from build123d import *

# Parameters (mm, degrees)
CUT_EXTRUDE1_DEPTH = 1.5


with BuildPart() as part:
    # Sketch1 → Revolve1 (revolve)
    with BuildSketch(Plane.XY):
        with BuildLine():
            Line((42.2, 0), (42.2, 1.61))
            Line((42.2, 1.61), (41.81, 2))
            Line((41.81, 2), (2.2, 2))
            Line((2.2, 2), (2.2, 3.8))
            Line((2.2, 3.8), (1.82, 3.8))
            ThreePointArc((1.82, 3.8), (0.762013659, 2.991755338), (0, 1.9))
            Line((0, 1.9), (0, 0))
            Line((0, 0), (42.2, 0))
        make_face()
    revolve(axis=Axis((42.2, 0, 0), (-1, 0, 0)))

    # Sketch2 → Cut-Extrude1 (cut)
    with BuildSketch(Plane.ZY):
        Polygon((-1.25, 0.721687836), (-1.25, -0.721687836), (0, -1.443375673), (1.25, -0.721687836), (1.25, 0.721687836), (0, 1.443375673), align=None)
    extrude(amount=-CUT_EXTRUDE1_DEPTH, mode=Mode.SUBTRACT)


solid = part.part
Model file for the job. Use its own axes, mm. A direction names the side the tool comes from. Give positions to 0.01 mm unless a question says otherwise; leave off trailing zeros. Order: outer loops, then holes, each group sorted by start corner. A loop starts at its lowest first (then second) coordinate and runs counter-clockwise, first axis right, second up. Notation, with made-up numbers: (89, 15.25) - (140, 15.25) arc R10 ccw to (140, 31.25) - close; hole circle Ø6 at (13, 46.5). An arc over 180 degrees is marked (long way). Write item = value, one per line. Start each with the question number.
1. Cut at B-B, the plane x = 18.5. List the corners of the cut face in (y, z), and give its area (3 significant figures).
2. Cut at C-C, the plane y = -2.5. List the corners of the cut face in (x, z), and give its area (3 significant figures).
3. Two-plate mould, pull along Z, no slides. Class faces 4 (the cylindrical face through (22, 0, 2)), 5 (the flat face through (42.2, 0, 0)), 6 (the flat face through (1, 0, 1.25)): pulls with the +Z half, pulls with the -Z half, needs draft (parallel to the pull), parting line crosses it, or undercut.
4. Probe line 1 along X through (y, z) = (-0.25, -0.75); line 2 along Z through (x, y) = (15.5, 0); line 3 along Z through (x, y) = (29.5, 1.75). List the from-to ranges inside material, lowest first.
5. Which spindle directions (+Z, -Z, +X, -X, +Y, -Y) get a long thin tool onto all of the face, cutting with end or side? Do faces 1 (the flat face through (2.2, -2, 2)), 2 (the cylindrical face through (2.007, -3.796, -0.167)), 3 (the flat face through (0.74, 1.088, -0.616)). Say none if no direction does.
6. Drop flat-ended pins along their axis: P1, Ø3, axis at x = 32.5, y = -0.5, coming from the +Z side; P2, Ø1.5, axis at x = 6.5, y = -2.5, coming from the +Z side; P3, Ø3, axis at x = 23.5, z = -2.5, coming from the +Y side. Give the stop position or say it passes through.
7. Cut at A-A, the plane y = 0. List the corners of the cut face in (x, z), and give its area (3 significant figures).
Taken from the geometry:
q1.outline = circle Ø4 at (0, 0)
q1.area = 12.6 mm²
q2.outline = (1.82, -2.86) - (2.2, -2.86) - (2.2, 2.86) - (1.82, 2.86) arc R3.53 ccw to start
q2.area = 8.04 mm²
q3.face_4 = parting line crosses it
q3.face_5 = needs draft
q3.face_6 = undercut
q4.line_1 = 1.5 to 42.2
q4.line_2 = -2 to 2
q4.line_3 = -0.97 to 0.97
q5.face_1 = +X
q5.face_2 = +X, -X
q5.face_3 = -X
q6.P1 = 2
q6.P2 = 0.97
q6.P3 = 1.73
q7.outline = (0, -1.9) arc R4.32 ccw to (1.82, -3.8) - (2.2, -3.8) - (2.2, -2) - (41.81, -2) - (42.2, -1.61) - (42.2, 1.61) - (41.81, 2) - (2.2, 2) - (2.2, 3.8) - (1.82, 3.8) arc R4.32 ccw to (0, 1.9) - (0, 1.25) - (1.5, 1.25) - (1.5, -1.25) - (0, -1.25) - close
q7.area = 170 mm²
